```python
from build123d import *

# Parameters (mm, degrees)
F1_DEPTH = 33
F3_DEPTH = 12
F5_DEPTH = 33.001


with BuildPart() as f1:
    # F0 (on Top) → F1 (new body)
    with BuildSketch(Plane.XY):
        with BuildLine():
            Line((-13, 27.037012), (13, 27.037012))
            ThreePointArc((13, 27.037012), (0, 30), (-13, 27.037012))
        make_face()
        with BuildLine():
            ThreePointArc((-13, -27.037012), (0, -30), (13, -27.037012))
            Line((13, -27.037012), (-13, -27.037012))
        make_face()
        with BuildLine():
            Line((13, -12), (6, -12))
            ThreePointArc((6, -12), (0, -18), (-6, -12))
            Line((-6, -12), (-13, -12))
            Line((-13, -12), (-13, -27.037012))
            Line((-13, -27.037012), (13, -27.037012))
            Line((13, -27.037012), (13, -12))
        make_face()
        with BuildLine():
            ThreePointArc((-6, -12), (0, -6), (6, -12))
            Line((6, -12), (13, -12))
            Line((13, -12), (13, 12))
            Line((13, 12), (6, 12))
            ThreePointArc((6, 12), (0, 6), (-6, 12))
            Line((-6, 12), (-13, 12))
            Line((-13, 12), (-13, -12))
            Line((-13, -12), (-6, -12))
        make_face()
        with BuildLine():
            Line((6, 12), (13, 12))
            Line((13, 12), (13, 27.037012))
            Line((13, 27.037012), (-13, 27.037012))
            Line((-13, 27.037012), (-13, 12))
            Line((-13, 12), (-6, 12))
            ThreePointArc((-6, 12), (0, 18), (6, 12))
        make_face()
    extrude(amount=F1_DEPTH)

    # F2 (on Top) → F3 (join)
    with BuildSketch(Plane.XY):
        with BuildLine():
            Line((-12.883144, 20), (22.36068, 20))
            ThreePointArc((22.36068, 20), (0, 30), (-22.36068, 20))
            Line((-22.36068, 20), (-12.883144, 20))
        make_face()
        with BuildLine():
            ThreePointArc((-22.36068, -20), (0, -30), (22.36068, -20))
            Line((22.36068, -20), (-12.883144, -20))
            Line((-12.883144, -20), (-22.36068, -20))
        make_face()
    extrude(amount=F3_DEPTH)

    # F4 (on face) → F5 (cut, through all)
    with BuildSketch(Plane.XY.offset(33)):
        Polygon((0, 36.60208), (0, 35.889369), (0, 33.03853), (0, -37.947364), (28.590711, -37.947364), (28.590711, 36.60208), align=None)
    extrude(amount=-F5_DEPTH, mode=Mode.SUBTRACT)


solid = f1.part
```
Input: part model. Units: mm. Frame: model coordinates. A direction names the side the tool comes from. Coordinates: 2 decimals unless noted, no trailing zeros. Write each loop counter-clockwise with the first axis right and the second up, starting at its lowest first coordinate (ties: lowest second). Pieces come first, ordered by that corner, then holes. Notation, with made-up numbers: (-32, -35.75) - (21, -35.75) arc R24 ccw to (21, -7.75) - close; hole circle Ø5 at (23, -10). An arc over 180 degrees is marked (long way). Put each result on its own line as item: value. Start each with the question number.
1) Cut plane A-A (x = -17.5). Return the cut outline in (y, z).
2) Contact query for flat-ended pins moving along their axis: pin 1 (2 mm diameter, centred on x = -14.5, z = 29.5, fed in from +Y); pin 2 (12 mm diameter, centred on y = 23, z = 20, fed in from -X); pin 3 (3 mm diameter, centred on x = -19, z = 7, fed in from +Y); pin 4 (3.5 mm diameter, centred on x = -17, y = -22.5, fed in from +Z). Output: stop coordinate, or through.
3) Cut plane C-C (x = -2). Return the cut outline in (y, z).
4) Mould query, pull axis Y, two halves, no side actions, for faces 1 (the face through (-7, 0, 33)), 2 (the face through (-6, -12, 16)). Classes: pulls with the +Y half, pulls with the -Y half, needs draft (parallel to the pull), parting line crosses it, or undercut.
5) Cut plane B-B (z = 18.5). Return the cut outline in (x, y), plus the area to 3 significant figures.
6) Cut plane D-D (y = 4). Return the cut outline in (x, z), plus the area to 3 significant figures.
7) Reachability of faces 3 (the face through (-17, -23, 12)), 4 (the face through (-18, -20, 6)), 5 (the face through (-6, 12, 16)) from +Z, -Z, +X, -X, +Y, -Y: full face, straight path, thin tool, end or side. Return the list, or none.
8) Ray query, L1, parallel to Y at x = -0.75, z = 6; L2, parallel to Y at x = -18.25, z = 7.5; L3, parallel to Z at x = -13.5, y = -21.5. Return the intervals inside material, ascending.
Resolved:
1. outline: (-24.37, 0) - (-20, 0) - (-20, 12) - (-24.37, 12) - close; (20, 0) - (24.37, 0) - (24.37, 12) - (20, 12) - close
2. pin 1: passes through
2. pin 2: stops at x = -13
2. pin 3: stops at y = 24.37
2. pin 4: stops at z = 12
3. outline: (-29.93, 0) - (-17.66, 0) - (-17.66, 33) - (-29.93, 33) - close; (-6.34, 0) - (6.34, 0) - (6.34, 33) - (-6.34, 33) - close; (17.66, 0) - (29.93, 0) - (29.93, 33) - (17.66, 33) - close
4. face 1: needs draft
4. face 2: undercut
5. outline: (-13, -27.04) arc R30 ccw to (0, -30) - (0, -18) arc R6 cw to (0, -6) - (0, 6) arc R6 cw to (0, 18) - (0, 30) arc R30 ccw to (-13, 27.04) - close
5. area: 642 mm2
6. outline: (-13, 0) - (0, 0) - (0, 33) - (-13, 33) - close
6. area: 429 mm2
7. face 3: +Z, -X, +Y, -Y
7. face 4: +Z, -Z, -X
7. face 5: +Z, -Z, +X
8. L1: y = -29.99 to -17.95, -6.05 to 6.05, 17.95 to 29.99
8. L2: y = -23.81 to -20, 20 to 23.81
8. L3: z = 0 to 12
